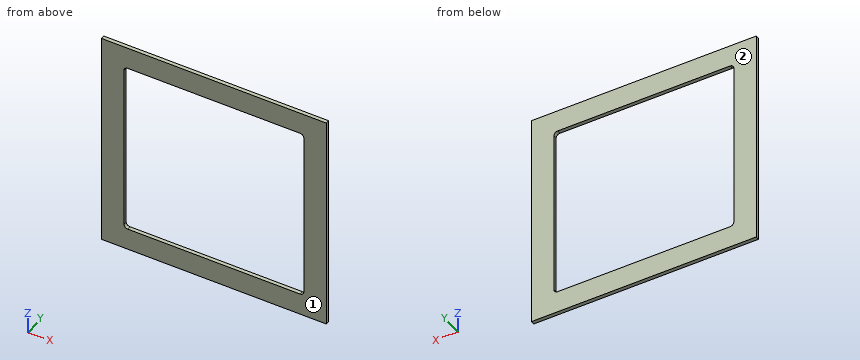
```python
from build123d import *

# Parameters (mm, degrees)
F0_W     = 600
F0_H     = 600
F1_DEPTH = 10


with BuildPart() as f1:
    # F0 (on Front) → F1 (new body)
    with BuildSketch(Plane.XZ):
        with Locations((300, 300)):
            Rectangle(F0_W, F0_H)
        with BuildLine():
            ThreePointArc((60, 530), (62.928932, 537.071068), (70, 540))
            Line((70, 540), (530, 540))
            ThreePointArc((530, 540), (537.071068, 537.071068), (540, 530))
            Line((540, 530), (540, 70))
            ThreePointArc((540, 70), (537.071068, 62.928932), (530, 60))
            Line((530, 60), (70, 60))
            ThreePointArc((70, 60), (62.928932, 62.928932), (60, 70))
            Line((60, 70), (60, 530))
        make_face(mode=Mode.SUBTRACT)
    extrude(amount=F1_DEPTH)


solid = f1.part
```
Input: part model. Units: mm. Frame: model coordinates. Face numbers are marked on the shaded views. Give positions to 0.01 mm unless a question says otherwise; leave off trailing zeros. Loops run counter-clockwise (first coordinate to the right, second up) from the corner with the lowest first, then second, coordinate; pieces in that order, holes last.
1) Section query A-A on y = -8. Return the cut outline in (x, z), and give its area (3 significant figures).
A:
outline: (0, 0) - (600, 0) - (600, 600) - (0, 600) - close; hole (60, 70) arc R10 ccw to (70, 60) - (530, 60) arc R10 ccw to (540, 70) - (540, 530) arc R10 ccw to (530, 540) - (70, 540) arc R10 ccw to (60, 530) - close
area: 130,000 mm2
2) Section query B-B on x = 256. Return the cut outline in (y, z).
A:
outline: (-10, 0) - (0, 0) - (0, 60) - (-10, 60) - close; (-10, 540) - (0, 540) - (0, 600) - (-10, 600) - close
3) Section query C-C on z = 250. Return the cut outline in (x, y).
A:
outline: (0, -10) - (60, -10) - (60, 0) - (0, 0) - close; (540, -10) - (600, -10) - (600, 0) - (540, 0) - close
4) Line query: L1, parallel to X at y = -8.5, z = 89.5. Output: solid intervals per line, ascending.
A:
L1: x = 0 to 60, 540 to 600
5) Mould query, pull axis Y, two halves, no side actions, for the marked faces 1 and 2. Classes: released by +Y, released by -Y, zero draft, split by the parting line, or undercut.
A:
face 1: released by -Y
face 2: released by +Y
